Design review of the part built by this model. Coordinates are the model's own, in mm. A direction names the side the tool comes from. Coordinates: 2 decimals unless noted, no trailing zeros. Order: outer loops, then holes, each group sorted by start corner. A loop starts at its lowest first (then second) coordinate and runs counter-clockwise, first axis right, second up. Notation, with made-up numbers: (62.25, -38.5) - (81.25, -38.5) arc R12 cw to (81.25, -18.5) - close; hole circle Ø6 at (-6, -21). An arc over 180 degrees is marked (long way). Write item = value, one per line. Start each with the question number.
```python
from build123d import *

# Parameters (mm, degrees)
F0_W     = 44.45
F0_H     = 6.35
F1_DEPTH = 4.064
F2_R     = 1.325099
F3_DEPTH = 25.4
F5_DEPTH = 25.4
F7_W     = 44.487826
F7_H     = 1.40328
F8_DEPTH = 12.7


with BuildPart() as f1:
    # F0 (on Front) → F1 (new body)
    with BuildSketch(Plane.XZ):
        Rectangle(F0_W, F0_H)
    extrude(amount=F1_DEPTH)

    # F2 (on face) → F3 (cut)
    with BuildSketch(Plane.XZ.offset(4.064)):
        with Locations((-18.36648, 0)):
            Circle(F2_R)
    extrude(amount=-F3_DEPTH, mode=Mode.SUBTRACT)

    # F2 (on face) → F5 (cut)
    with BuildSketch(Plane.XZ.offset(4.064)):
        with Locations((-18.36648, 0)):
            Circle(F2_R)
    extrude(amount=-F5_DEPTH, mode=Mode.SUBTRACT)

    # F6: F1 across plane


with BuildPart() as f1_1:
    add(f1.part)
    add(f1.part.mirror(Plane.YZ), mode=Mode.INTERSECT)

    # F7 (on face) → F8 (join)
    with BuildSketch(Plane.XZ.offset(4.064)):
        with Locations((0, -2.45779)):
            Rectangle(F7_W, F7_H)
    extrude(amount=F8_DEPTH)


solid = f1_1.part
```
Item 1: For faces 1 (the flat face through (0, -4.064, 1)), 2 (the cylindrical face through (-19.69, -2.06, 0.06)), list the 3-axis set-ups (+Z, -Z, +X, -X, +Y, -Y) from which the entire face can be reached by the end or side of a thin tool; tool diameter is ignored.
Item 2: Mouldability with a two-part tool opening along Z and no side actions: class faces 3 (the flat face through (0, -2, 3.175)), 4 (the cylindrical face through (19.69, -2.06, 0.06)), 5 (the flat face through (0, -2, -3.175)) as +Z half, -Z half, draft (parallel to the pull), parting line (faces both ways), or undercut.
Item 3: Add section A-A on z = 0. Give the boundary of the cut face in (x, y) (3 decimals), plus the area to 3 significant figures.
Item 4: Add section C-C on y = -2.25. Give the boundary of the cut face in (x, z) (3 decimals), plus the area to 3 significant figures.
Item 5: For P1, Ø3.5, axis at y = -2.5, z = -0.5, coming from the +X side (3 decimals); P2, Ø1.5, axis at x = 3.5, y = -10, coming from the -Z side; P3, Ø6.5, axis at x = 0.5, y = -12, coming from the +Z side, all flat-tipped, find the tip position at first contact; note any pin that passes through.
Item 6: Add section B-B on x = 10. Give the boundary of the cut face in (y, z) (3 decimals), plus the area to 3 significant figures.
Item 7: For line 1 (X direction, y = -2, z = 1) (3 decimals); line 2 (Z direction, x = -18.5, y = -5); line 3 (Y direction, x = 13, z = -1.25), list the stretches that pass through material, from the lowest coordinate up.
Item 8: Add section D-D on y = -13. Give the boundary of the cut face in (x, z), plus the area to 3 significant figures.
Worked out:
q1.face_1 = +Z, +X, -X, -Y
q1.face_2 = +Y, -Y
q2.face_3 = +Z half
q2.face_4 = undercut
q2.face_5 = -Z half
q3.outline = (-22.225, -4.064) - (-19.692, -4.064) - (-19.692, 0) - (-22.225, 0) - close; (-17.041, -4.064) - (17.041, -4.064) - (17.041, 0) - (-17.041, 0) - close; (19.692, -4.064) - (22.225, -4.064) - (22.225, 0) - (19.692, 0) - close
q3.area = 159 mm2
q4.outline = (-22.225, -3.175) - (22.225, -3.175) - (22.225, 3.175) - (-22.225, 3.175) - close; hole circle Ø2.65 at (-18.366, 0); hole circle Ø2.65 at (18.366, 0)
q4.area = 271 mm2
q5.P1 = 22.225
q5.P2 = -3.16
q5.P3 = -1.76
q6.outline = (-16.764, -3.159) - (-4.064, -3.159) - (-4.064, -3.175) - (0, -3.175) - (0, 3.175) - (-4.064, 3.175) - (-4.064, -1.756) - (-16.764, -1.756) - close
q6.area = 43.6 mm2
q7.line_1 = -22.225 to -19.236, -17.497 to 17.497, 19.236 to 22.225
q7.line_2 = -3.16 to -1.76
q7.line_3 = -4.06 to 0
q8.outline = (-22.24, -3.16) - (22.24, -3.16) - (22.24, -1.76) - (-22.24, -1.76) - close
q8.area = 62.4 mm2
